from build123d import *

# Parameters (mm, degrees)
SKETCH1_R           = 1.5
BOSS_EXTRUDE1_DEPTH = 6


with BuildPart() as part:
    # Sketch1 → Boss-Extrude1 (new body)
    with BuildSketch(Plane(origin=(0, 0, 0), x_dir=(0, 0, -1), z_dir=(1, 0, 0))):
        Polygon((50, 0), (70, 0), (70, 4), (85.592625509, 47.729644272), (109.224105862, 34.086002729), (131.486359031, 60.617122922), (131.486359031, 65.598790277), (95.255608124, 96), (56.74353499, 96), (44.099407436, 80.931315562), (57.225143451, 65.28867251), (50.426653107, 57), (0, 57), (0, 51), (45.505365409, 51), (25, 26), (0, 26), (0, 20), (25, 20), (50, 2), align=None)
        with Locations((85, 55)):
            Circle(SKETCH1_R, mode=Mode.SUBTRACT)
        Polygon((30.059592338, 23.750495981), (61.737302817, 61.50252125), (80.310098668, 50.779512566), (64.343122912, 6), (54.713058978, 6), align=None, mode=Mode.SUBTRACT)
        with BuildLine():
            Line((59.541380939, 90), (51.931851172, 80.931315562))
            Line((51.931851172, 80.931315562), (61.09679395, 70.00896208))
            Line((61.09679395, 70.00896208), (63.350780176, 72.757006533))
            ThreePointArc((63.350780176, 72.757006533), (65.090587223, 74.687947655), (67.001946929, 76.449244407))
            ThreePointArc((67.001946929, 76.449244407), (71.228443087, 76.079473907), (70.858672587, 71.852977749))
            ThreePointArc((70.858672587, 71.852977749), (68.147022251, 69.141327413), (65.947441117, 66))
            Line((65.947441117, 66), (81.968911087, 56.75))
            ThreePointArc((81.968911087, 56.75), (86.75, 58.031088913), (88.031088913, 53.25))
            Line((88.031088913, 53.25), (107.864016281, 41.799454045))
            Line((107.864016281, 41.799454045), (125.486359031, 62.800944328))
            Line((125.486359031, 62.800944328), (93.071786719, 90))
            Line((93.071786719, 90), (59.541380939, 90))
        make_face(mode=Mode.SUBTRACT)
        with BuildLine():
            ThreePointArc((67.966128343, 75.300177743), (64.699822257, 72.033871657), (62.0503268, 68.25))
            ThreePointArc((62.0503268, 68.25), (62.599364905, 66.200961894), (64.648403011, 66.75))
            ThreePointArc((64.648403011, 66.75), (66.997955587, 70.105508828), (69.894491172, 73.002044413))
            ThreePointArc((69.894491172, 73.002044413), (70.079376423, 75.115292493), (67.966128343, 75.300177743))
        make_face(mode=Mode.SUBTRACT)
    boss_extrude1 = extrude(amount=BOSS_EXTRUDE1_DEPTH)

    # Sketch2 → Tap Drill for M3 Tap1 (revolve, cut)
    with BuildSketch(Plane(origin=(3, 0, -60), x_dir=(0, 0, -1), z_dir=(1, 0, 0))):
        Polygon((0, 0), (0, 10.751075774), (1.25, 10), (1.25, 0), align=None)
    tap_drill_for_m3_tap1 = revolve(axis=Axis((3, -6.35, -60), (0, 1, 0)), mode=Mode.SUBTRACT)

    # Mirror1: Boss-Extrude1, Tap Drill for M3 Tap1 across plane
    add(boss_extrude1.mirror(Plane.XY))
    add(tap_drill_for_m3_tap1.mirror(Plane.XY), mode=Mode.SUBTRACT)


solid = part.part
Geometry check sheet. Reference: the model listing, model coordinates, mm. A direction names the side the tool comes from. Coordinates: 2 decimals unless noted, no trailing zeros. Order: outer loops, then holes, each group sorted by start corner. A loop starts at its lowest first (then second) coordinate and runs counter-clockwise, first axis right, second up. Notation, with made-up numbers: (-15.75, -28) - (-8.75, -28) arc R16 ccw to (-8.75, 3) - close; hole circle Ø2 at (5, -22.75). An arc over 180 degrees is marked (long way). Answer in a Markdown table with one row per item. Add a question column.
1) Material ranges on line 1 along Z through (x, y) = (3, 1.8); line 2 along X through (y, z) = (4.5, 60); line 3 along Y through (x, z) = (4.15, 49), recorded low to high. Write a range as [from, to].
2) Cross-section at A-A, the plane z = -21.5. Record the cut outline in (x, y), then the cut area to 3 significant figures.
3) Gauge pin test, flat ends, axial feed: P1, Ø2, axis at x = 1.5, y = 37.5, coming from the +Z side; P2, Ø2, axis at x = 4, z = -97, coming from the +Y side; P3, Ø0.6, axis at x = 4, y = 1, coming from the +Z side. Record the tip position at first contact, or that the pin passes through.
4) Set-up check for faces 1 (the flat face through (2.958, 11.126, 37.325)), 2 (the flat face through (2.958, 47.166, -120.199)), 3 (the flat face through (2.958, 61.44, -73.846)): record each of +Z, -Z, +X, -X, +Y, -Y from which the full face is reachable in a straight line by a thin tool's end or side.
Check result:
| question | item | result |
|---|---|---|
| 1 | line 1 | z = [-70, -61.25], [-58.75, -50], [50, 58.75], [61.25, 70] |
| 1 | line 2 | x = [0, 1.75], [4.25, 6] |
| 1 | line 3 | y = [2.72, 10.11], [46.32, 57], [75.09, 86.77] |
| 2 | outline | (0, 20) - (6, 20) - (6, 26) - (0, 26) - close; (0, 51) - (6, 51) - (6, 57) - (0, 57) - close |
| 2 | area | 72.0 mm² |
| 3 | P1 | stops at z = 112.93 |
| 3 | P2 | stops at y = 95.38 |
| 3 | P3 | stops at z = 70 |
| 4 | face 1 | +X, -X, -Y |
| 4 | face 2 | -Z, +X, -X, -Y |
| 4 | face 3 | +X, -X |
